```python
from build123d import *

# Parameters (mm, degrees)
SKETCH1_R           = 1.5
SKETCH1_R_2         = 2
SKETCH1_R_3         = 8
BOSS_EXTRUDE1_DEPTH = 3


with BuildPart() as part:
    # Sketch1 → Boss-Extrude1 (new body)
    with BuildSketch(Plane.XY):
        with BuildLine():
            Line((5, 28), (5, 25))
            ThreePointArc((5, 25), (10.857864376, 10.857864376), (25, 5))
            Line((25, 5), (28, 5))
            ThreePointArc((28, 5), (33, 0), (28, -5))
            Line((28, -5), (25, -5))
            ThreePointArc((25, -5), (10.857864376, -10.857864376), (5, -25))
            Line((5, -25), (5, -28))
            ThreePointArc((5, -28), (0, -33), (-5, -28))
            Line((-5, -28), (-5, -25))
            ThreePointArc((-5, -25), (-10.857864376, -10.857864376), (-25, -5))
            Line((-25, -5), (-28, -5))
            ThreePointArc((-28, -5), (-33, 0), (-28, 5))
            Line((-28, 5), (-25, 5))
            ThreePointArc((-25, 5), (-10.857864376, 10.857864376), (-5, 25))
            Line((-5, 25), (-5, 28))
            ThreePointArc((-5, 28), (0, 33), (5, 28))
        make_face()
        with Locations((0, 28)):
            Circle(SKETCH1_R, mode=Mode.SUBTRACT)
        with Locations((28, 0)):
            Circle(SKETCH1_R, mode=Mode.SUBTRACT)
        with Locations((0, -28)):
            Circle(SKETCH1_R, mode=Mode.SUBTRACT)
        with Locations((-28, 0)):
            Circle(SKETCH1_R, mode=Mode.SUBTRACT)
        with Locations((0, -11.313708499)):
            Circle(SKETCH1_R_2, mode=Mode.SUBTRACT)
        with Locations((-11.313708499, 0)):
            Circle(SKETCH1_R_2, mode=Mode.SUBTRACT)
        with Locations((0, 11.313708499)):
            Circle(SKETCH1_R_2, mode=Mode.SUBTRACT)
        with Locations((11.313708499, 0)):
            Circle(SKETCH1_R_2, mode=Mode.SUBTRACT)
        Circle(SKETCH1_R_3, mode=Mode.SUBTRACT)
    extrude(amount=BOSS_EXTRUDE1_DEPTH)


solid = part.part
```
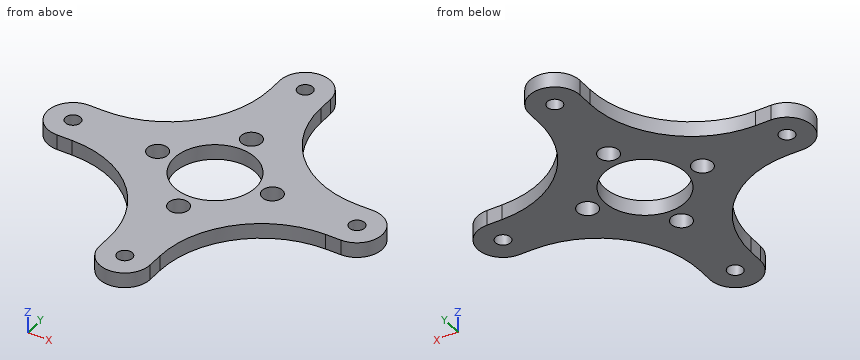
The model under review builds one solid part; all positions refer to its coordinate system, in mm. Give positions to 0.01 mm unless a question says otherwise; leave off trailing zeros. Write each loop counter-clockwise with the first axis right and the second up, starting at its lowest first coordinate (ties: lowest second). Pieces come first, ordered by that corner, then holes.
(1) For P1, Ø1, axis at y = 25.5, z = 1.5, coming from the +X side; P2, Ø1.5, axis at x = -27, z = 1, coming from the -Y side; P3, Ø0.9, axis at x = 27, z = 1, coming from the +Y side, all flat-tipped, find the tip position at first contact; note any pin that passes through.
(2) Consider section C-C, the plane z = 2.2. Give the number of separate pieces and of enclosed holes in the cut face, and give its area (3 significant figures).
(3) To check wall thickness, follow L1, parallel to Y at x = 0, z = 1; L2, parallel to Y at x = 0.5, z = 0.25; L3, parallel to Y at x = 28, z = 0.9. State the ranges of each line that lie inside material, in increasing order.
(4) Consider section A-A, the plane y = 0. Give the boundary of the cut face in (x, z), and give its area (3 significant figures).
(5) Consider section D-D, the plane x = 15.5. Give the boundary of the cut face in (y, z), and give its area (3 significant figures).
Returned:
1. P1: stops at x = 5
1. P2: stops at y = -5
1. P3: stops at y = 5
2. separate pieces: 1
2. enclosed holes: 9
2. area: 1,240 mm2
3. L1: y = -33 to -29.5, -26.5 to -13.31, -9.31 to -8, 8 to 9.31, 13.31 to 26.5, 29.5 to 33
3. L2: y = -32.97 to -29.41, -26.59 to -13.25, -9.38 to -7.98, 7.98 to 9.38, 13.25 to 26.59, 29.41 to 32.97
3. L3: y = -5 to -1.5, 1.5 to 5
4. outline: (-33, 0) - (-29.5, 0) - (-29.5, 3) - (-33, 3) - close; (-26.5, 0) - (-13.31, 0) - (-13.31, 3) - (-26.5, 3) - close; (-9.31, 0) - (-8, 0) - (-8, 3) - (-9.31, 3) - close; (8, 0) - (9.31, 0) - (9.31, 3) - (8, 3) - close; (13.31, 0) - (26.5, 0) - (26.5, 3) - (13.31, 3) - close; (29.5, 0) - (33, 0) - (33, 3) - (29.5, 3) - close
4. area: 108 mm2
5. outline: (-7.4, 0) - (7.4, 0) - (7.4, 3) - (-7.4, 3) - close
5. area: 44.4 mm2
